```python
from build123d import *

# Parameters (mm, degrees)
FILLET_1_R = 3


with BuildPart() as part:
    # 草图1 → Revolve 292 (revolve)
    with BuildSketch(Plane.XY, mode=Mode.PRIVATE) as revolve_292_sk:
        Polygon((0, 0), (20, 0), (20, 12), (13, 12), (13, 72), (7, 107), (0, 107), align=None)
    revolve(revolve_292_sk.sketch.rotate(Axis((0, 0, 0), (0, 1, 0)), 90), axis=Axis((0, 0, 0), (0, 1, 0)))

    # 圆角1
    fillet_1_edges = [part.edges().sort_by_distance(p)[0] for p in [
        (0, 72, 13),
    ]]
    fillet(fillet_1_edges, radius=FILLET_1_R)


solid = part.part
```
Read the model definition and answer for the solid it produces. Units are mm, in the model's axes. A direction names the side the tool comes from. Give positions to 0.01 mm unless a question says otherwise; leave off trailing zeros. Loops run counter-clockwise (first coordinate to the right, second up) from the corner with the lowest first, then second, coordinate; pieces in that order, holes last.
Item 1: For faces 1 (the cylindrical face through (7.91, 42.291, 10.316)), 2 (the flat face through (0, 0, 0)), determine the directions among +Z, -Z, +X, -X, +Y, -Y from which every point of the face is accessible in a straight line to the end or side of a thin tool.
Item 2: The part is cut by section C-C (y = 8). Write down the section's boundary in (x, z).
Item 3: Each of these flat-tipped pins is pushed along its axis until it touches: pin 1 Ø6 at (x, y) = (1, 40) entering from +Z; pin 2 Ø8 at (x, y) = (-5.5, 86.5) entering from +Z; pin 3 Ø2 at (x, z) = (-14, -7.5) entering from +Y; pin 4 Ø6 at (x, z) = (7.5, -4) entering from +Y. Where does it stop, or does it pass through?
Item 4: The part is cut by section B-B (x = 14). Write down the section's boundary in (y, z), and give its area (3 significant figures).
Item 5: The part is cut by section A-A (y = 93). Write down the section's boundary in (x, z).
Item 6: Find the intervals of material crossed by line 1 along Y through (x, z) = (-1, 14.5); line 2 along X through (y, z) = (99.5, -2); line 3 along Z through (x, y) = (-11, 76), in increasing order.
Taken from the geometry:
1. face 1: +Y
1. face 2: +Z, -Z, +X, -X, -Y
2. outline: circle Ø40 at (0, 0)
3. pin 1: stops at z = 13
3. pin 2: stops at z = 10.68
3. pin 3: stops at y = 12
3. pin 4: stops at y = 107
4. outline: (0, -14.28) - (12, -14.28) - (12, 14.28) - (0, 14.28) - close
4. area: 343 mm2
5. outline: circle Ø18.8 at (0, 0)
6. line 1: y = 0 to 12
6. line 2: x = -8.04 to 8.04
6. line 3: z = -5.54 to 5.54
